from build123d import *

# Parameters (mm, degrees)
SKETCH2_R = 2.5


with BuildPart() as part:
    # Sweep1: sweep along a path in Sketch1
    with BuildLine(Plane.XY) as sweep1_path:
        Line((210, -73.885714286), (157.459682683, -73.885714286))
        ThreePointArc((157.459682683, -73.885714286), (154.190143217, -73.336117012), (151.279989747, -71.747736622))
        Line((151.279989747, -71.747736622), (62.720010253, -2.137977664))
        ThreePointArc((62.720010253, -2.137977664), (59.809856783, -0.549597274), (56.540317317, 0))
        Line((56.540317317, 0), (-56.540317317, 0))
        ThreePointArc((-56.540317317, 0), (-59.809856783, -0.549597274), (-62.720010253, -2.137977664))
        Line((-62.720010253, -2.137977664), (-151.279989747, -71.747736622))
        ThreePointArc((-151.279989747, -71.747736622), (-154.190143217, -73.336117012), (-157.459682683, -73.885714286))
        Line((-157.459682683, -73.885714286), (-210, -73.885714286))
    # Sketch2 → Sweep1 (sweep)
    with BuildSketch(Plane(origin=(210, -73.885714286, 0), x_dir=(0, 0, -1), z_dir=(1, 0, 0))):
        with Locations((0, -0.042530313)):
            Circle(SKETCH2_R)
    sweep(path=sweep1_path.line)


solid = part.part
CAD build for the part. Positions are in the model's coordinates, mm. Coordinates: 2 decimals unless noted, no trailing zeros. Loops run counter-clockwise (first coordinate to the right, second up) from the corner with the lowest first, then second, coordinate; pieces in that order, holes last. Notation, with made-up numbers: (4.25, 77) - (15.25, 77) arc R14 cw to (15.25, 95) - close; hole circle Ø5 at (62.5, 0.25). An arc over 180 degrees is marked (long way). Write item = value, one per line. Start each with the question number.
Q1. Flat gauge pins, fed straight in: pin 1 Ø1 at (y, z) = (-37.5, 1.5) entering from -X; pin 2 Ø1.5 at (x, z) = (-13.5, -1) entering from +Y. Where does each tip first touch, or does it go through?
Q2. Drill centre lines: L1, parallel to X at y = -54.5, z = -0.9; L2, parallel to X at y = -24, z = -0.7; L3, parallel to Y at x = 16, z = -0.5. Where is each one in solid material? Low to high.
Q3. Cut at B-B, the plane x = 4. List the corners of the cut face in (y, z).
Q4. Cut at A-A, the plane z = 0. List the corners of the cut face in (x, y).
Computed:
q1.pin_1 = -111.7
q1.pin_2 = 2.44
q2.L1 = -133.04 to -125.49, 125.49 to 133.04
q2.L2 = -94.35 to -86.58, 86.58 to 94.35
q2.L3 = -2.49 to 2.41
q3.outline = circle Ø5 at (-0.04, 0)
q4.outline = (-210, -76.43) - (-157.46, -76.43) arc R12.54 ccw to (-149.71, -73.75) - (-61.15, -4.14) arc R7.46 cw to (-56.54, -2.54) - (56.54, -2.54) arc R7.46 cw to (61.15, -4.14) - (149.71, -73.75) arc R12.54 ccw to (157.46, -76.43) - (210, -76.43) - (210, -71.43) - (157.46, -71.43) arc R7.54 cw to (152.8, -69.82) - (64.24, -0.21) arc R12.46 ccw to (56.54, 2.46) - (-56.54, 2.46) arc R12.46 ccw to (-64.24, -0.21) - (-152.8, -69.82) arc R7.54 cw to (-157.46, -71.43) - (-210, -71.43) - close
